Here's how the part is built. I have some questions about the finished solid (model axes, mm). A direction names the side the tool comes from. Round coordinates to 2 decimals unless told otherwise and drop trailing zeros. Order: outer loops, then holes, each group sorted by start corner. A loop starts at its lowest first (then second) coordinate and runs counter-clockwise, first axis right, second up. Notation, with made-up numbers: (0.5, -13.5) - (19.5, -13.5) arc R8 ccw to (19.5, -7.5) - close; hole circle Ø1 at (-24.75, 4). An arc over 180 degrees is marked (long way). Answer as a JSON object with one key per item and string values.
```python
from build123d import *

# Parameters (mm, degrees)
F1_DEPTH = 12.7
F0_R     = 1.63195
F2_DEPTH = 19.05
F3_R     = 1.35255
F4_DEPTH = 25.4
F5_DEPTH = 6.35
F6_R     = 1.35255
F7_DEPTH = 25.4
F8_R     = 1.35255
F9_DEPTH = 12.701


with BuildPart() as f1:
    # F0 (on Front) → F1 (new body)
    with BuildSketch(Plane.XZ):
        with BuildLine():
            ThreePointArc((-3.175, 18.7835533113), (-12.2967221242, -14.5496778315), (19.05, 0))
            ThreePointArc((19.05, 0), (14.5496778315, 12.2967221242), (3.175, 18.7835533113))
            Line((3.175, 18.7835533113), (3.175, 8.9802561211))
            ThreePointArc((3.175, 8.9802561211), (7.7771299333, 5.499261314), (9.525, 0))
            ThreePointArc((9.525, 0), (-5.499261314, -7.7771299333), (-3.175, 8.9802561211))
            Line((-3.175, 8.9802561211), (-3.175, 18.7835533113))
        make_face()
        with BuildLine():
            Line((3.175, 8.9802561211), (3.175, 18.7835533113))
            ThreePointArc((3.175, 18.7835533113), (0, 19.05), (-3.175, 18.7835533113))
            Line((-3.175, 18.7835533113), (-3.175, 8.9802561211))
            ThreePointArc((-3.175, 8.9802561211), (0, 9.525), (3.175, 8.9802561211))
        make_face()
    extrude(amount=F1_DEPTH)

    # F0 (on Front) → F2 (join)
    with BuildSketch(Plane.XZ):
        with BuildLine():
            Line((3.175, -6.35), (3.175, 8.9802561211))
            ThreePointArc((3.175, 8.9802561211), (0, 9.525), (-3.175, 8.9802561211))
            Line((-3.175, 8.9802561211), (-3.175, -6.35))
            Line((-3.175, -6.35), (3.175, -6.35))
        make_face()
        Circle(F0_R, mode=Mode.SUBTRACT)
        with BuildLine():
            ThreePointArc((9.525, 0), (7.7771299333, 5.499261314), (3.175, 8.9802561211))
            Line((3.175, 8.9802561211), (3.175, -6.35))
            Line((3.175, -6.35), (-3.175, -6.35))
            Line((-3.175, -6.35), (-3.175, 8.9802561211))
            ThreePointArc((-3.175, 8.9802561211), (-5.499261314, -7.7771299333), (9.525, 0))
        make_face()
    extrude(amount=F2_DEPTH)

    # F3 (on Right) → F4 (cut)
    with BuildSketch(Plane.YZ):
        with Locations((-15.875, 0)):
            Circle(F3_R)
    extrude(amount=-F4_DEPTH, mode=Mode.SUBTRACT)

    # F0 (on Front) → F5 (cut)
    with BuildSketch(Plane.XZ):
        with BuildLine():
            ThreePointArc((-3.175, 18.7835533113), (0, 19.05), (3.175, 18.7835533113))
            Line((3.175, 18.7835533113), (3.175, 19.7523720562))
            Line((3.175, 19.7523720562), (-3.175, 19.7523720562))
            Line((-3.175, 19.7523720562), (-3.175, 18.7835533113))
        make_face()
        with BuildLine():
            Line((3.175, 8.9802561211), (3.175, 18.7835533113))
            ThreePointArc((3.175, 18.7835533113), (0, 19.05), (-3.175, 18.7835533113))
            Line((-3.175, 18.7835533113), (-3.175, 8.9802561211))
            ThreePointArc((-3.175, 8.9802561211), (0, 9.525), (3.175, 8.9802561211))
        make_face()
        with BuildLine():
            Line((3.175, -6.35), (3.175, 8.9802561211))
            ThreePointArc((3.175, 8.9802561211), (0, 9.525), (-3.175, 8.9802561211))
            Line((-3.175, 8.9802561211), (-3.175, -6.35))
            Line((-3.175, -6.35), (3.175, -6.35))
        make_face()
        Circle(F0_R, mode=Mode.SUBTRACT)
    extrude(amount=F5_DEPTH, mode=Mode.SUBTRACT)

    # F6 (on face) → F7 (cut)
    with BuildSketch(Plane(origin=(0, -6.35, 0), x_dir=(-1, 0, 0), z_dir=(0, 1, 0))):
        with Locations((0, 11.43)):
            Circle(F6_R)
    extrude(amount=-F7_DEPTH, mode=Mode.SUBTRACT)

    # F8 (on face) → F9 (cut, through all)
    with BuildSketch(Plane.XY.offset(-6.35)):
        with Locations((0, -3.175)):
            Circle(F8_R)
    extrude(amount=-F9_DEPTH, mode=Mode.SUBTRACT)


solid = f1.part
```
1. Imagine slicing it at B-B (z = 11.43). List the corners of the cut face in (x, y) for me (3 decimals).
Responses:
{"outline": "(-15.24, -12.7) - (-1.353, -12.7) - (-1.353, -6.35) - (-3.175, -6.35) - (-3.175, 0) - (-15.24, 0) - close; (1.353, -12.7) - (15.24, -12.7) - (15.24, 0) - (3.175, 0) - (3.175, -6.35) - (1.353, -6.35) - close"}
2. Imagine slicing it at A-A (x = 0). List the corners of the cut face in (y, z) for me (3 decimals), plus the area to 3 significant figures.
Responses:
{"outline": "(-19.05, -9.525) - (-12.7, -9.525) - (-12.7, -19.05) - (-4.528, -19.05) - (-4.528, -6.35) - (-6.35, -6.35) - (-6.35, -1.632) - (-19.05, -1.632) - close; (-19.05, 1.632) - (-6.35, 1.632) - (-6.35, 10.077) - (-12.7, 10.077) - (-12.7, 9.525) - (-19.05, 9.525) - close; (-12.7, 12.783) - (-6.35, 12.783) - (-6.35, 19.05) - (-12.7, 19.05) - close; (-1.822, -19.05) - (0, -19.05) - (0, -6.35) - (-1.822, -6.35) - close", "area": "351 mm2"}
3. If I drill on L1, parallel to Z at x = 0, y = -16 (3 decimals); L2, parallel to Y at x = -5, z = 0; L3, parallel to Z at x = 0, y = -9, over which ranges is the centre line in solid material (lowest first)? Write a range as [from, to].
Responses:
{"L1": "[-9.525, -1.632], [1.632, 9.525]", "L2": "[-19.05, -17.23], [-14.52, 0]", "L3": "[-19.05, -1.63], [1.63, 10.08], [12.78, 19.05]"}
4. For P1, Ø1, axis at y = -11, z = -5.5, coming from the +X side; P2, Ø3, axis at y = -3, z = 10, coming from the -X side; P3, Ø2, axis at x = 13.5, z = 3.5, coming from the -Y side; P4, Ø2.5, axis at x = 0, z = 0, coming from the -Y side (1 decimal), each with a flat end and sliding along its axis, tell me the tip position at first contact or that it passes through.
Responses:
{"P1": "x = 18.38", "P2": "x = -17.05", "P3": "y = -12.7", "P4": "through"}
5. Imagine slicing it at C-C (y = -7.25). List the corners of the cut face in (x, z) for me (3 decimals), plus the area to 3 significant figures.
Responses:
{"outline": "circle Ø38.1 at (0, 0); hole circle Ø3.264 at (0, 0); hole circle Ø2.705 at (0, 11.43)", "area": "1,130 mm2"}
6. Imagine slicing it at D-D (z = -8). List the corners of the cut face in (x, y) for me (3 decimals), plus the area to 3 significant figures.
Responses:
{"outline": "(-17.289, -12.7) - (-5.17, -12.7) - (-5.17, -19.05) - (5.17, -19.05) - (5.17, -12.7) - (17.289, -12.7) - (17.289, 0) - (-17.289, 0) - close; hole circle Ø2.705 at (0, -3.175)", "area": "499 mm2"}
7. Thinking about a two-plate mould opening in Z: for faces 4 (the face through (-9, -12.7, -4)), 5 (the face through (1.508, -12.611, -0.625)), 6 (the face through (0, -5, -6.35)), which applies, pulls with the +Z half, pulls with the -Z half, needs draft (parallel to the pull), parting line crosses it, or undercut?
Responses:
{"face 4": "needs draft", "face 5": "undercut", "face 6": "pulls with the +Z half"}
8. For faces 1 (the face through (-0.293, -4.495, -12.612)), 2 (the face through (3.175, -3, 6)), 3 (the face through (-5.16, -14.585, 0.406)), which set-ups out of +Z, -Z, +X, -X, +Y, -Y let a thin tool reach every point of the face, with its end or its side?
Responses:
{"face 1": "+Z, -Z", "face 2": "+Z, +Y", "face 3": "-X"}
